from build123d import *

# Parameters (mm, degrees)
SKETCH1_R           = 10
BOSS_EXTRUDE1_DEPTH = 5.4
BOSS_EXTRUDE2_DEPTH = 5.4
CIRPATTERN1_COUNT   = 24
SKETCH3_R           = 12.65
SKETCH3_R_2         = 12
CUT_EXTRUDE1_DEPTH  = 6
CUT_EXTRUDE2_DEPTH  = 6
SKETCH5_R           = 1.7
CUT_EXTRUDE3_DEPTH  = 6
BOSS_EXTRUDE3_DEPTH = 5.4


with BuildPart() as part:
    # Sketch1 → Boss-Extrude1 (new body)
    with BuildSketch(Plane.XY):
        Circle(SKETCH1_R)
    extrude(amount=BOSS_EXTRUDE1_DEPTH)

    # Sketch2 → Boss-Extrude2 (add)
    with BuildSketch(Plane.XY):
        with BuildLine():
            Line((0, 12.65), (-0.9, 9.959417654))
            ThreePointArc((-0.9, 9.959417654), (0, 10), (0.9, 9.959417654))
            Line((0.9, 9.959417654), (0, 12.65))
        make_face()
    boss_extrude2 = extrude(amount=BOSS_EXTRUDE2_DEPTH)

    # CirPattern1: Boss-Extrude2 ×24 about axis
    cirpattern1_axis = Axis((0, 0, 0), (0, 0, 1))
    for i in range(1, CIRPATTERN1_COUNT):
        add(boss_extrude2.rotate(cirpattern1_axis, i * 360 / CIRPATTERN1_COUNT))

    # Sketch3 → Cut-Extrude1 (cut)
    with BuildSketch(Plane.XY):
        Circle(SKETCH3_R)
        Circle(SKETCH3_R_2, mode=Mode.SUBTRACT)
    extrude(amount=CUT_EXTRUDE1_DEPTH, mode=Mode.SUBTRACT)

    # Sketch4 → Cut-Extrude2 (cut)
    with BuildSketch(Plane.XY):
        with BuildLine():
            Line((0, 0), (0, -12))
            ThreePointArc((0, -12), (11.769423365, 2.341083864), (-4.592201188, 11.08655439))
            Line((-4.592201188, 11.08655439), (-3.826834324, 9.238795325))
            Line((-3.826834324, 9.238795325), (0, 0))
        make_face()
    extrude(amount=CUT_EXTRUDE2_DEPTH, mode=Mode.SUBTRACT)

    # Sketch5 → Cut-Extrude3 (cut)
    with BuildSketch(Plane.XY):
        Circle(SKETCH5_R)
    extrude(amount=CUT_EXTRUDE3_DEPTH, mode=Mode.SUBTRACT)

    # Sketch6 → Boss-Extrude3 (add)
    with BuildSketch(Plane.XY):
        with BuildLine():
            Line((-4.32, 9.438795325), (-4.32, 10.9))
            Line((-4.32, 10.9), (0, 10.9))
            Line((0, 10.9), (0, 14.7))
            Line((0, 14.7), (7, 14.7))
            Line((7, 14.7), (7, 10.9))
            Line((7, 10.9), (11, 10.9))
            Line((11, 10.9), (11, -9.1))
            Line((11, -9.1), (7, -9.1))
            Line((7, -9.1), (7, -12))
            Line((7, -12), (0, -12))
            Line((0, -12), (0, -1.65))
            ThreePointArc((0, -1.65), (1.472580529, 0.744316187), (-1.328564272, 0.978476865))
            Line((-1.328564272, 0.978476865), (-4.32, 9.438795325))
        make_face()
    extrude(amount=BOSS_EXTRUDE3_DEPTH)


solid = part.part
Input: part model. Units: mm. Frame: model coordinates. A direction names the side the tool comes from. Coordinates: 2 decimals unless noted, no trailing zeros. Order: outer loops, then holes, each group sorted by start corner. A loop starts at its lowest first (then second) coordinate and runs counter-clockwise, first axis right, second up. Notation, with made-up numbers: M 26.25,-10 L 56.25,-10 A9 ccw 56.25,7 Z; hole C -33.5,43 d10. An arc over 180 degrees is marked long. Answer in a Markdown table with one row per item.
(1) Section query A-A, the plane y = 9.75. Output: boundary loops of the cut face in (x, z), plus the area to 3 significant figures.
Numbers:
| item | result |
|---|---|
| outline | M -6.08,0 L -4.96,0 L -4.96,5.4 L -6.08,5.4 Z; M -4.32,0 L 11,0 L 11,5.4 L -4.32,5.4 Z |
| area | 88.8 mm^2 |
(2) Contact query for flat-ended pins moving along their axis: pin 1 Ø1.6 at (y, z) = (10, 3) entering from -X; pin 2 Ø1 at (y, z) = (11.5, 2) entering from +X; pin 3 Ø1.9 at (y, z) = (13.5, 2) entering from -X. Output: stop coordinate, or through.
Numbers:
| item | result |
|---|---|
| pin 1 | stops at x = -6.19 |
| pin 2 | stops at x = 7 |
| pin 3 | stops at x = 0 |
(3) Material intervals for line 1 (X direction, y = 0, z = 1.65); line 2 (Y direction, x = -9.75, z = 2.05); line 3 (X direction, y = 11.25, z = 2.2), sorted ascending. Write a range as [from, to].
Numbers:
| item | result |
|---|---|
| line 1 | x = [-12, -1.7], [1.65, 11] |
| line 2 | y = [-6.08, -4.96], [-3.42, 3.42], [4.96, 6.08] |
| line 3 | x = [0, 7] |
(4) Section query B-B, the plane x = 9.25. Output: boundary loops of the cut face in (y, z).
Numbers:
| item | result |
|---|---|
| outline | M -9.1,0 L 10.9,0 L 10.9,5.4 L -9.1,5.4 Z |
(5) Section query C-C, the plane y = 12.5. Output: boundary loops of the cut face in (x, z), plus the area to 3 significant figures.
Numbers:
| item | result |
|---|---|
| outline | M 0,0 L 7,0 L 7,5.4 L 0,5.4 Z |
| area | 37.8 mm^2 |
(6) Access query for faces 1 (the flat face through (-7.35, 8.15, 2.66)), 2 (the flat face through (-10.964, 0.564, 2.662)), 3 (the flat face through (7, -11, 3)). Directions: +Z, -Z, +X, -X, +Y, -Y. A direction counts if a zero-diameter tool reaches every point of the face in a straight line with its end or side. Return the directions, or none.
Numbers:
| item | result |
|---|---|
| face 1 | +Z, -Z, +Y |
| face 2 | +Z, -Z, -X |
| face 3 | +Z, -Z, +X, -Y |
(7) Draft query along Y for faces 4 (the flat face through (-3.382, -10.445, 2.662)), 5 (the flat face through (11, 1, 3)), 6 (the flat face through (-9.243, -5.977, 2.662)). Return one class per face: pulls with the +Y half, pulls with the -Y half, needs draft (parallel to the pull), parting line crosses it, or undercut.
Numbers:
| item | result |
|---|---|
| face 4 | pulls with the -Y half |
| face 5 | needs draft |
| face 6 | undercut |
